Verification items for this drawing (mm, ordinates from the low corner). A direction names the side the tool comes from. Round coordinates to 2 decimals unless told otherwise and drop trailing zeros. Loops run counter-clockwise (first coordinate to the right, second up) from the corner with the lowest first, then second, coordinate; pieces in that order, holes last. Notation, with made-up numbers: (26, 24.25) -> (74, 24.25) arc R20 ccw to (74, 33.25) -> close; hole circle Ø9 at (-30.75, -22). An arc over 180 degrees is marked (long way). One line per item, written item: value. Start each with the question number.
1. Release check for a two-part mould opening along Y. For the marked faces 1, 2 and 3 record: +Y half, -Y half, draft (parallel to the pull), parting line (faces both ways), or undercut.
2. Go/stop test with flat-tipped pins: pin 1 (1 mm diameter, centred on x = 6.5, z = 1, fed in from -Y); pin 2 (0.6 mm diameter, centred on y = 10, z = 0.5, fed in from +X); pin 3 (1 mm diameter, centred on y = 14, z = 1, fed in from -X). Record where each tip stops, or that it passes through.
3. Set-up check for the marked faces 4, 5, 6, 7 and 8: record each of +Z, -Z, +X, -X, +Y, -Y from which the full face is reachable in a straight line by a thin tool's end or side.
4. Material ranges on L1, parallel to Y at x = 16.25, z = 2.15; L2, parallel to X at y = 11, z = 3.35; L3, parallel to Y at x = 14.75, z = 1.45, recorded low to high.
5. Cross-section at A-A on z = 2.8. Record the cut outline in (x, y).
6. Cross-section at C-C on x = 17.5. Record the cut outline in (y, z), then the cut area to 3 significant figures.
7. Cross-section at D-D on z = 1.6. Record the cut outline in (x, y), then the cut area to 3 significant figures.
8. Cross-section at B-B on y = 9. Record the cut outline in (x, z), then the cut area to 3 significant figures.
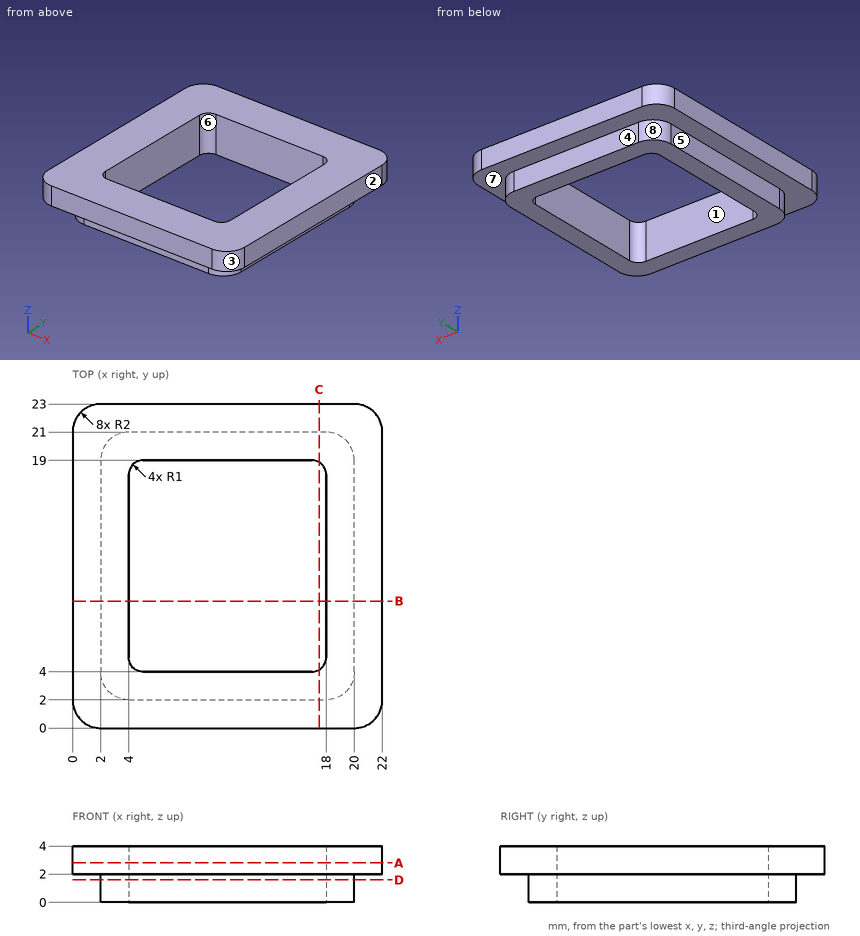
Taken from the geometry:
1. face 1: undercut
1. face 2: draft
1. face 3: -Y half
2. pin 1: stops at y = 2
2. pin 2: stops at x = 20
2. pin 3: stops at x = 2
3. face 4: -Z, +X, -X, +Y
3. face 5: -Z, -X, +Y, -Y
3. face 6: +Z, -Z
3. face 7: -Z
3. face 8: -Z, -X, +Y
4. L1: y = 0 to 4, 19 to 23
4. L2: x = 0 to 4, 18 to 22
4. L3: y = 2 to 4, 19 to 21
5. outline: (0, 2) arc R2 ccw to (2, 0) -> (20, 0) arc R2 ccw to (22, 2) -> (22, 21) arc R2 ccw to (20, 23) -> (2, 23) arc R2 ccw to (0, 21) -> close; hole (4, 5) arc R1 ccw to (5, 4) -> (17, 4) arc R1 ccw to (18, 5) -> (18, 18) arc R1 ccw to (17, 19) -> (5, 19) arc R1 ccw to (4, 18) -> close
6. outline: (0, 2) -> (2, 2) -> (2, 0) -> (4.13, 0) -> (4.13, 4) -> (0, 4) -> close; (18.87, 0) -> (21, 0) -> (21, 2) -> (23, 2) -> (23, 4) -> (18.87, 4) -> close
6. area: 25.1 mm2
7. outline: (2, 4) arc R2 ccw to (4, 2) -> (18, 2) arc R2 ccw to (20, 4) -> (20, 19) arc R2 ccw to (18, 21) -> (4, 21) arc R2 ccw to (2, 19) -> close; hole (4, 5) arc R1 ccw to (5, 4) -> (17, 4) arc R1 ccw to (18, 5) -> (18, 18) arc R1 ccw to (17, 19) -> (5, 19) arc R1 ccw to (4, 18) -> close
7. area: 129 mm2
8. outline: (0, 2) -> (2, 2) -> (2, 0) -> (4, 0) -> (4, 4) -> (0, 4) -> close; (18, 0) -> (20, 0) -> (20, 2) -> (22, 2) -> (22, 4) -> (18, 4) -> close
8. area: 24.0 mm2
